Input: part model. Units: mm. Frame: model coordinates. Face numbers are marked on the shaded views. A direction names the side the tool comes from. Give positions to 0.01 mm unless a question says otherwise; leave off trailing zeros. Loops run counter-clockwise (first coordinate to the right, second up) from the corner with the lowest first, then second, coordinate; pieces in that order, holes last. Notation, with made-up numbers: M 31.5,42 L 85.5,42 A13 cw 85.5,64 Z; hole C 76.5,83.5 d8. An arc over 180 degrees is marked long. Answer as a JSON object with one key per item and string values. Group by question number.
```python
from build123d import *

# Parameters (mm, degrees)
BOSS_EXTRUDE1_DEPTH     = 20
CUT_EXTRUDE3_DEPTH      = 50.867148527
CUT_EXTRUDE3_DEPTH_BACK = 50.867148527
CUT_EXTRUDE4_DEPTH      = 51.602966037
CUT_EXTRUDE4_DEPTH_BACK = 51.602966037


with BuildPart() as part:
    # Sketch1 → Boss-Extrude1 (new body)
    with BuildSketch(Plane.XY):
        Polygon((0, 0), (35, 0), (46.642135624, -11.642135624), (53.713203436, -4.571067812), (43.106601718, 6.035533906), (38.535533906, 1.464466094), (35, 5), (0, 5), align=None)
    extrude(amount=BOSS_EXTRUDE1_DEPTH)

    # Sketch2 → Cut-Extrude3 (cut, two sides: drawn at the far end of the back side and taken through both)
    with BuildSketch(Plane(origin=(29.142135624, -29.142135624, 0), x_dir=(0, 0, -1), z_dir=(0.7071067811865479, -0.7071067811865471, 0)).offset(-CUT_EXTRUDE3_DEPTH_BACK)):
        Polygon((-14, 135.155901118), (-14, 34.748737342), (-14, 32.748737342), (-12, 32.748737342), (-12, 30.748737342), (-8, 30.748737342), (-8, 32.792627222), (-6, 32.792627222), (-6, 34.748737342), (-6, 135.155901118), (-6, 335.970228672), (-14, 335.970228672), align=None)
    extrude(amount=CUT_EXTRUDE3_DEPTH + CUT_EXTRUDE3_DEPTH_BACK, mode=Mode.SUBTRACT)

    # Sketch4 → Cut-Extrude4 (cut, two sides: drawn at the far end of the back side and taken through both)
    with BuildSketch(Plane(origin=(24.571067812, 24.571067812, 0), x_dir=(0, 0, -1), z_dir=(0.7071067811865477, 0.7071067811865475, 0)).offset(-CUT_EXTRUDE4_DEPTH_BACK)):
        with BuildLine():
            Line((89.549076457, 16.380836563), (0, -38.283901601))
            ThreePointArc((0, -38.283901601), (-9.934867623, -41.207301416), (-20, -38.769890621))
            Line((-20, -38.769890621), (-112.098466498, 11.480911975))
            Line((-112.098466498, 11.480911975), (-107.001191072, -198.288248186))
            Line((-107.001191072, -198.288248186), (94.646351884, -193.388323598))
            Line((94.646351884, -193.388323598), (89.549076457, 16.380836563))
        make_face()
    extrude(amount=CUT_EXTRUDE4_DEPTH + CUT_EXTRUDE4_DEPTH_BACK, mode=Mode.SUBTRACT)


solid = part.part
```
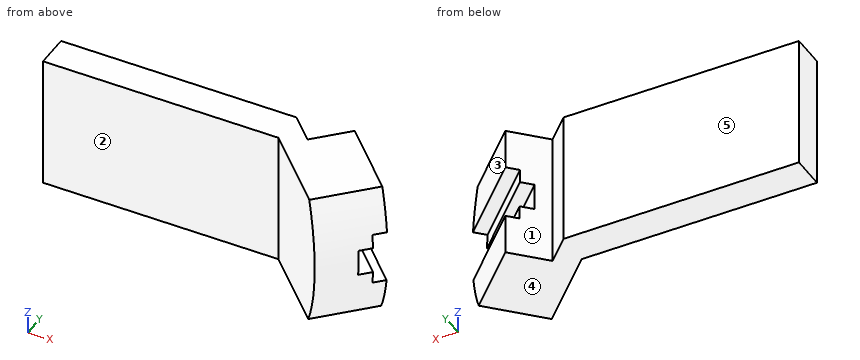
1. Reachability of the marked faces 4 and 5 from +Z, -Z, +X, -X, +Y, -Y: full face, straight path, thin tool, end or side. Return the list, or none.
2. Section A-A (z = 17.75). Output: boundary loops of the cut face in (x, y), then the cut area to 3 significant figures.
3. Mould query, pull axis X, two halves, no side actions, for the marked faces 1, 2 and 3. Classes: pulls with the +X half, pulls with the -X half, needs draft (parallel to the pull), parting line crosses it, or undercut.
4. Section B-B (y = 0.5). Output: boundary loops of the cut face in (x, z).
5. First-contact query: P1, Ø5, axis at x = 23, z = 10, coming from the +Y side; P2, Ø3, axis at x = 10, z = 3, coming from the -Y side. Flat tips, straight axial feed; report the tip coordinate or a pass-through.
6. Section C-C (x = 29). Output: boundary loops of the cut face in (y, z).
7. Section D-D (z = 2.25). Output: boundary loops of the cut face in (x, y), then the cut area to 3 significant figures.
8. Material intervals for L1, parallel to Y at x = 17, z = 6.5; L2, parallel to X at y = 4, z = 13; L3, parallel to X at y = 2, z = 6.5, sorted ascending.
Geometry results:
{
 "1": {"face 4": "-Z, +X, -X, +Y, -Y", "face 5": "+Z, -Z, -X, +Y"},
 "2": {"outline": "M 0,0 L 35,0 L 45.66,-10.66 L 52.73,-3.59 L 43.11,6.04 L 38.54,1.46 L 35,5 L 0,5 Z", "area": "323 mm2"},
 "3": {"face 1": "undercut", "face 2": "needs draft", "face 3": "pulls with the +X half"},
 "4": {"outline": "M 0,0 L 48.64,0 L 48.64,6 L 45.88,6 L 45.88,8 L 42.99,8 L 42.99,12 L 45.81,12 L 45.81,14 L 48.64,14 L 48.64,20 L 0,20 Z"},
 "5": {"P1": "y = 5", "P2": "y = 0"},
 "6": {"outline": "M 0,0 L 5,0 L 5,20 L 0,20 Z"},
 "7": {"outline": "M 0,0 L 35,0 L 45.41,-10.41 L 52.48,-3.34 L 43.11,6.04 L 38.54,1.46 L 35,5 L 0,5 Z", "area": "319 mm2"},
 "8": {"L1": "0 to 5", "L2": "0 to 36, 41.07 to 42.31", "L3": "0 to 38, 39.07 to 44.38"}
}
